Check sheet for the modelled part. Datum: model origin and axes. Units: mm. A direction names the side the tool comes from. Coordinates: 2 decimals unless noted, no trailing zeros. Order: outer loops, then holes, each group sorted by start corner. A loop starts at its lowest first (then second) coordinate and runs counter-clockwise, first axis right, second up.
1. Set-up check for faces 5 (the flat face through (1, 161.925, 0)), 6 (the flat face through (-1.588, 86, 30)), 7 (the flat face through (0, 111.125, -6)): record each of +Z, -Z, +X, -X, +Y, -Y from which the full face is reachable in a straight line by a thin tool's end or side.
2. Gauge pin test, flat ends, axial feed: pin 1 Ø1 at (x, y) = (12.5, 78) entering from +Z (3 decimals); pin 2 Ø1.9 at (x, z) = (1.5, 18) entering from -Y; pin 3 Ø1.9 at (x, z) = (1.5, 6.5) entering from -Y (3 decimals). Record the tip position at first contact, or that the pin passes through.
3. Cross-section at B-B (y = 44). Count the separate pieces of the cut face and the enclosed holes in it, then the cut area to 3 significant figures.
4. Thickness scan on line 1 (Z direction, x = 0, y = 57) (3 decimals); line 2 (Z direction, x = 0, y = 0.6); line 3 (Y direction, x = 21, z = -17.5) (3 decimals). Record the ranges inside material, lowest first.
5. Cross-section at A-A (x = 49.5). Enter the section's corners in (y, z) (3 decimals).
6. Draft check along Y on faces 1 (the flat face through (-36.512, 85, 30)), 2 (the flat face through (1.588, 85, 30)), 3 (the flat face through (52, 85, 31.75)), 4 (the flat face through (-6, 111.125, 0)). Enter one of: released by +Y, released by -Y, zero draft, split by the parting line, or undercut.
```python
from build123d import *

# Parameters (mm, degrees)
F0_R     = 25.4
F0_R_2   = 3.175
F0_R_3   = 1.5875
F1_DEPTH = 9.525
F2_W     = 114.3
F2_H     = 63.5
F3_DEPTH = 152.4
F5_DEPTH = 3.175
F6_DEPTH = 0.79375
F7_DEPTH = 101.6


with BuildPart() as f1:
    # F0 (on Front) → F1 (new body)
    with BuildSketch(Plane.XZ):
        Circle(F0_R)
        with Locations((0, -16.66875)):
            Circle(F0_R_2, mode=Mode.SUBTRACT)
        with Locations((-16.66875, 0)):
            Circle(F0_R_2, mode=Mode.SUBTRACT)
        with Locations((0, -5.55625)):
            Circle(F0_R_2, mode=Mode.SUBTRACT)
        with Locations((-5.55625, 0)):
            Circle(F0_R_3, mode=Mode.SUBTRACT)
        with Locations((0, 5.55625)):
            Circle(F0_R_2, mode=Mode.SUBTRACT)
        with Locations((0, 16.66875)):
            Circle(F0_R_2, mode=Mode.SUBTRACT)
        with Locations((-16.66875, 0)):
            Circle(F0_R_2)
        with Locations((0, 16.66875)):
            Circle(F0_R_2)
    extrude(amount=-F1_DEPTH)

    # F2 (on face) → F3 (join)
    with BuildSketch(Plane(origin=(0, 9.525, 0), x_dir=(-1, 0, 0), z_dir=(0, 1, 0))):
        Rectangle(F2_W, F2_H)
    extrude(amount=F3_DEPTH)

    # F4 (on face) → F5 (cut)
    with BuildSketch(Plane.XY.offset(31.75)):
        with BuildLine():
            ThreePointArc((-1.5875, 34.925), (0, 33.3375), (1.5875, 34.925))
            Line((1.5875, 34.925), (1.5875, 136.525))
            ThreePointArc((1.5875, 136.525), (0, 138.1125), (-1.5875, 136.525))
            Line((-1.5875, 136.525), (-1.5875, 34.925))
        make_face()
        with BuildLine():
            Line((11.1125, 136.525), (11.1125, 34.925))
            ThreePointArc((11.1125, 34.925), (12.7, 33.3375), (14.2875, 34.925))
            Line((14.2875, 34.925), (14.2875, 136.525))
            ThreePointArc((14.2875, 136.525), (12.7, 138.1125), (11.1125, 136.525))
        make_face()
        with BuildLine():
            Line((23.8125, 136.525), (23.8125, 34.925))
            ThreePointArc((23.8125, 34.925), (25.4, 33.3375), (26.9875, 34.925))
            Line((26.9875, 34.925), (26.9875, 136.525))
            ThreePointArc((26.9875, 136.525), (25.4, 138.1125), (23.8125, 136.525))
        make_face()
        with BuildLine():
            Line((36.5125, 136.525), (36.5125, 34.925))
            ThreePointArc((36.5125, 34.925), (38.1, 33.3375), (39.6875, 34.925))
            Line((39.6875, 34.925), (39.6875, 136.525))
            ThreePointArc((39.6875, 136.525), (38.1, 138.1125), (36.5125, 136.525))
        make_face()
        with BuildLine():
            Line((-23.8125, 34.925), (-23.8125, 136.525))
            ThreePointArc((-23.8125, 136.525), (-25.4, 138.1125), (-26.9875, 136.525))
            Line((-26.9875, 136.525), (-26.9875, 34.925))
            ThreePointArc((-26.9875, 34.925), (-25.4, 33.3375), (-23.8125, 34.925))
        make_face()
        with BuildLine():
            Line((-11.1125, 34.925), (-11.1125, 136.525))
            ThreePointArc((-11.1125, 136.525), (-12.7, 138.1125), (-14.2875, 136.525))
            Line((-14.2875, 136.525), (-14.2875, 34.925))
            ThreePointArc((-14.2875, 34.925), (-12.7, 33.3375), (-11.1125, 34.925))
        make_face()
        with BuildLine():
            Line((-39.6875, 136.525), (-39.6875, 34.925))
            ThreePointArc((-39.6875, 34.925), (-38.1, 33.3375), (-36.5125, 34.925))
            Line((-36.5125, 34.925), (-36.5125, 136.525))
            ThreePointArc((-36.5125, 136.525), (-38.1, 138.1125), (-39.6875, 136.525))
        make_face()
    extrude(amount=-F5_DEPTH, mode=Mode.SUBTRACT)

    # F0 (on Front) → F6 (cut)
    with BuildSketch(Plane.XZ):
        with Locations((0, 16.66875)):
            Circle(F0_R_2)
        with Locations((-16.66875, 0)):
            Circle(F0_R_2)
    extrude(amount=-F6_DEPTH, mode=Mode.SUBTRACT)

    # F7 (cut): faces of the model
    f7_faces = [f1.faces().sort_by_distance(p)[0] for p in [
        (0, 9.525, 5.55625),
        (-5.55625, 9.525, 0),
        (0, 9.525, -5.55625),
        (0, 9.525, -16.66875),
    ]]
    extrude(f7_faces, amount=-F7_DEPTH, mode=Mode.SUBTRACT)


solid = f1.part
```
Data:
1. face 5: +Z, -Z, +X, -X, +Y
1. face 6: +Z
1. face 7: -Y
2. pin 1: stops at z = 28.575
2. pin 2: stops at y = 0.79
2. pin 3: stops at y = 111.125
3. separate pieces: 1
3. enclosed holes: 4
3. area: 7,080 mm2
4. line 1: z = -31.75 to -19.844, -13.494 to -8.731, -2.381 to 2.381, 8.731 to 28.575
4. line 2: z = -25.4 to -19.84, -13.49 to -8.73, -2.38 to 2.38, 8.73 to 13.49, 19.84 to 25.4
4. line 3: y = 9.525 to 161.925
5. outline: (9.525, -31.75) - (161.925, -31.75) - (161.925, 31.75) - (9.525, 31.75) - close
6. face 1: undercut
6. face 2: undercut
6. face 3: zero draft
6. face 4: released by -Y
